Read the model definition and answer for the solid it produces. Units are mm, in the model's axes. A direction names the side the tool comes from. Coordinates: 2 decimals unless noted, no trailing zeros. Loops run counter-clockwise (first coordinate to the right, second up) from the corner with the lowest first, then second, coordinate; pieces in that order, holes last. Notation, with made-up numbers: (-32.5, -35) -> (-11.5, -35) arc R31 cw to (-11.5, -5) -> close; hole circle Ø6 at (-22, -40). An arc over 180 degrees is marked (long way). Answer as a JSON object with one key per item and string values. Group by question number.
Q1. The part is cut by section D-D on y = 5. Write down the section's boundary in (x, z).
Q2. The part is cut by section B-B on y = 28. Write down the section's boundary in (x, z), and give its area (3 significant figures).
Q3. Each of these flat-tipped pins is pushed along its axis until it touches: P1, Ø8, axis at x = 4, z = 5.5, coming from the +Y side; P2, Ø12, axis at y = 34.5, z = -1, coming from the -X side; P3, Ø4.5, axis at y = 36.83, z = -7.69, coming from the +X side. Where does it stop, or does it pass through?
Q4. For faces 1 (the flat face through (-2, 0.2, 0)), 2 (the cylindrical face through (21.088, 24.533, 1.366)), 3 (the cylindrical face through (16.328, 10.257, 6.502)), determine the directions among +Z, -Z, +X, -X, +Y, -Y from which every point of the face is accessible in a straight line to the end or side of a thin tool.
Q5. The part is cut by section A-A on z = 0. Write down the section's boundary in (x, y).
Q6. Determine the mould class of faces 4 (the flat face through (5, 0, 18.3)), 5 (the flat face through (14.3, 16, 0)), 6 (the cylindrical face through (-2.22, -1.929, -13.503)), 7 (the cylindrical face through (16.3, 22.4, -18.1)) for opening direction Z: released by +Z, released by -Z, zero draft, split by the parting line, or undercut.
Q7. Straight lines are drawn through the part: line 1 along Z through (x, y) = (17.5, 24); line 2 along X through (y, z) = (29, -10); line 3 along Y through (x, z) = (2, -12). For each, find the intervals that lie inside material, in ascending order. Write a range as [from, to].
Q8. The part is cut by section C-C on z = -13. Write down the section's boundary in (x, y).
from build123d import *

# Parameters (mm, degrees)
EXTRUDE_1_DEPTH      = 40.6
EXTRUDE_1_DEPTH_BACK = 4
SKETCH_1_W           = 36.6
SKETCH_1_H           = 36.6
SKETCH_2_W           = 32.6
SKETCH_2_H           = 36.6
CUT_EXTRUDE_1_DEPTH  = 40.4
SKETCH_3_R           = 6.15
SKETCH_3_R_2         = 1.35
CUT_EXTRUDE_5_DEPTH  = 36.6
FILLET_2_R           = 2
SKETCH_7_R           = 1.6
CUT_EXTRUDE_6_DEPTH  = 10
CUT_EXTRUDE_8_DEPTH  = 10
FILLET_5_R           = 3
FILLET_6_R           = 3
SKETCH_17_R          = 7.2
EXTRUDE_2_DEPTH      = 5.5
SKETCH_18_R          = 6.3
CUT_EXTRUDE_9_DEPTH  = 5.5


with BuildPart() as part:
    # 草图1 → 凸台-拉伸1 (new, two sides: drawn at the far end of the back side and taken through both)
    with BuildSketch(Plane(origin=(0, 0, 0), x_dir=(1, 0, 0), z_dir=(0, 1, 0)).offset(-EXTRUDE_1_DEPTH_BACK)):
        Rectangle(SKETCH_1_W, SKETCH_1_H)
    extrude(amount=EXTRUDE_1_DEPTH + EXTRUDE_1_DEPTH_BACK)

    # 草图2 → 切除-拉伸1 (cut)
    with BuildSketch(Plane(origin=(0, 40.6, 0), x_dir=(1, 0, 0), z_dir=(0, 1, 0))):
        with Locations((-2, 0)):
            Rectangle(SKETCH_2_W, SKETCH_2_H)
    extrude(amount=-CUT_EXTRUDE_1_DEPTH, mode=Mode.SUBTRACT)

    # 草图3 → 切除-拉伸5 (cut)
    with BuildSketch(Plane(origin=(18.3, 0, 0), x_dir=(0, 0, -1), z_dir=(1, 0, 0))):
        with Locations((0, 30.682903148)):
            Circle(SKETCH_3_R)
        with Locations((-7.691951836, 36.832903148)):
            Circle(SKETCH_3_R_2)
        with Locations((7.691951836, 36.832903148)):
            Circle(SKETCH_3_R_2)
        with Locations((-15.529977583, 23.257044321)):
            Circle(SKETCH_3_R_2)
        with Locations((15.529977583, 23.257044321)):
            Circle(SKETCH_3_R_2)
        with Locations((7.745235234, 9.85104245)):
            Circle(SKETCH_3_R_2)
        with Locations((-7.790018794, 9.85104245)):
            Circle(SKETCH_3_R_2)
    extrude(amount=-CUT_EXTRUDE_5_DEPTH, mode=Mode.SUBTRACT)

    # 圆角2
    fillet_2_edges = [part.edges().sort_by_distance(p)[0] for p in [
        (16.3, 40.6, -18.3),
        (16.3, 40.6, 18.3),
    ]]
    fillet(fillet_2_edges, radius=FILLET_2_R)

    # 草图7 → 切除-拉伸6 (cut)
    with BuildSketch(Plane(origin=(0, -4, 0), x_dir=(-1, 0, 0), z_dir=(0, -1, 0))):
        with Locations(Location((1.606935512, 12.025, 0), (0, 0, 90))):
            Circle(SKETCH_7_R)
        with Locations(Location((10.106572894, 12.103513479, 0), (0, 0, 90))):
            Circle(SKETCH_7_R)
        with Locations(Location((10.106572894, -12.103513479, 0), (0, 0, 270))):
            Circle(SKETCH_7_R)
        with Locations(Location((1.606935512, -12.025, 0), (0, 0, 270))):
            Circle(SKETCH_7_R)
    extrude(amount=-CUT_EXTRUDE_6_DEPTH, mode=Mode.SUBTRACT)

    # 草图12 → 切除-拉伸8 (cut)
    with BuildSketch(Plane(origin=(18.3, 0, 0), x_dir=(0, 0, -1), z_dir=(1, 0, 0))):
        Polygon((-17.589988792, 23.257044321), (-11.626385684, 36.832903148), (-9.971575423, 40.6), (-18.3, 40.6), (-18.3, 23.257044321), align=None)
        Polygon((18.3, 23.257044321), (18.3, 40.6), (9.971575423, 40.6), (11.626385684, 36.832903148), (17.589988792, 23.257044321), align=None)
    extrude(amount=-CUT_EXTRUDE_8_DEPTH, mode=Mode.SUBTRACT)

    # 圆角5
    # the kernel refuses this fillet: 3 mm, written as the material it takes off along each edge
    with BuildSketch(Plane(origin=(23.145069229, 23.257044321, 18.3), x_dir=(0, -1, 0), z_dir=(-1, 0, 0))) as fillet_5_piece_1:
        with BuildLine():
            CenterArc((1.938027692, -3), FILLET_5_R, 90, 40.241386347)
            Line((0, -0.710011208), (-0.038760554, -0.664211432))
            ThreePointArc((-0.038760554, -0.664211432), (-0.06, -0.355005604), (-0.06, 0))
            Line((-0.06, 0), (0, 0.06))
            Line((0, 0.06), (1.938027692, 0.06))
            Line((1.938027692, 0.06), (1.938027692, 0))
        make_face()
    extrude(amount=13.690138458, mode=Mode.SUBTRACT)

    # 圆角6
    # the kernel refuses this fillet: 3 mm, written as the material it takes off along each edge
    with BuildSketch(Plane(origin=(23.145069229, 23.257044321, -18.3), x_dir=(0, -1, 0), z_dir=(-1, 0, 0))) as fillet_6_piece_1:
        with BuildLine():
            CenterArc((1.938027692, 3), FILLET_6_R, 229.758613653, 40.241386347)
            Line((0, 0.710011208), (-0.038760554, 0.664211432))
            ThreePointArc((-0.038760554, 0.664211432), (-0.06, 0.355005604), (-0.06, 0))
            Line((-0.06, 0), (0, -0.06))
            Line((0, -0.06), (1.938027692, -0.06))
            Line((1.938027692, -0.06), (1.938027692, 0))
        make_face()
    extrude(amount=13.690138458, mode=Mode.SUBTRACT)

    # 草图17 → 凸台-拉伸2 (add)
    with BuildSketch(Plane(origin=(18.3, 0, 0), x_dir=(0, 0, -1), z_dir=(1, 0, 0))):
        with Locations((0, 30.682903148)):
            Circle(SKETCH_17_R)
    extrude(amount=EXTRUDE_2_DEPTH)

    # 草图18 → 切除-拉伸9 (cut)
    with BuildSketch(Plane(origin=(23.8, 0, 0), x_dir=(0, 0, -1), z_dir=(1, 0, 0))):
        with Locations((0, 30.682903148)):
            Circle(SKETCH_18_R)
    extrude(amount=-CUT_EXTRUDE_9_DEPTH, mode=Mode.SUBTRACT)


solid = part.part
Final values:
{
 "1": {"outline": "(14.3, -18.3) -> (18.3, -18.3) -> (18.3, 18.3) -> (14.3, 18.3) -> close"},
 "2": {"outline": "(14.3, -15.51) -> (18.3, -15.51) -> (18.3, -6.68) -> (23.8, -6.68) -> (23.8, -5.7) -> (18.3, -5.7) -> (18.3, -5.53) -> (14.3, -5.53) -> close; (14.3, 5.53) -> (18.3, 5.53) -> (18.3, 5.7) -> (23.8, 5.7) -> (23.8, 6.68) -> (18.3, 6.68) -> (18.3, 15.51) -> (14.3, 15.51) -> close", "area": "90.6 mm2"},
 "3": {"P1": "stops at y = 0.2", "P2": "stops at x = 14.3", "P3": "stops at x = 18.3"},
 "4": {"face 1": "+Z, -Z, -X, +Y", "face 2": "+X", "face 3": "+X, -X"},
 "5": {"outline": "(-18.3, -4) -> (18.3, -4) -> (18.3, 23.48) -> (23.8, 23.48) -> (23.8, 24.38) -> (18.3, 24.38) -> (18.3, 24.53) -> (14.3, 24.53) -> (14.3, 0.2) -> (-18.3, 0.2) -> close; (14.3, 36.83) -> (18.3, 36.83) -> (18.3, 36.98) -> (23.8, 36.98) -> (23.8, 37.88) -> (18.3, 37.88) -> (18.3, 40.6) -> (14.3, 40.6) -> close"},
 "6": {"face 4": "released by +Z", "face 5": "zero draft", "face 6": "undercut", "face 7": "released by -Z"},
 "7": {"line 1": "z = [-17.26, -16.66], [-14.4, 14.4], [16.66, 17.26]", "line 2": "x = [14.3, 18.3]", "line 3": "y = [-4, 0.2]"},
 "8": {"outline": "(-18.3, -4) -> (-11.43, -4) -> (-11.43, 0.2) -> (-18.3, 0.2) -> close; (-8.78, -4) -> (-2.88, -4) -> (-2.88, 0.2) -> (-8.78, 0.2) -> close; (-0.34, -4) -> (18.3, -4) -> (18.3, 33.71) -> (14.3, 33.71) -> (14.3, 0.2) -> (-0.34, 0.2) -> close"}
}
